Autodesk Inventor part; units mm, degrees
ref_plane "YZ Plane" through (0, 0, 0) normal (1, 0, 0) x (0, 1, 0)
ref_plane "XZ Plane" through (0, 0, 0) normal (0, 1, 0) x (-1, 0, 0)
ref_plane "XY Plane" through (0, 0, 0) normal (0, 0, 1) x (1, 0, 0)
sketch "Sketch1" plane through (0, 0, 0) normal (0, 1, 0) x (-1, 0, 0)
  line L0 (3.175, -63.5) -> (-3.175, -63.5)
  line L1 (-3.175, -63.5) -> (-3.175, 63.5)
  line L2 (-3.175, 63.5) -> (3.175, 63.5)
  line L3 (3.175, 63.5) -> (3.175, -63.5)
  line L4 (3.175, -63.5) -> (-3.175, 63.5) construction
  line L5 (-3.175, -63.5) -> (3.175, 63.5) construction
  circle A0 centre (0, 60.325) radius 2.1082
  circle A1 centre (0, -60.325) radius 2.1082
  point P0 (0, 0)
  dimension "d0" = 6.35
  dimension "d1" = 127
  dimension "d2" = 4.2164
  dimension "d3" = 4.2164
  dimension "d4" = 3.175
  dimension "d5" = 3.175
  dimension "d6" = 3.175
  dimension "d7" = 3.175
extrude "Extrusion1" add sketch "Sketch1" along normal blind 6.35
fillet "Fillet1" radius 1.5875 4 edges at (3.175, 0, 0) (-3.175, 0, 0) (3.175, 6.35, 0) (-3.175, 6.35, 0)
fillet "Fillet2" radius 0.7937 16 edges at (0, 6.35, -63.5) (-2.71, 5.885, -63.5) (-3.175, 3.175, -63.5) (-2.71, 0.465, -63.5) (0, 0, -63.5) (2.71, 0.465, -63.5) (3.175, 3.175, -63.5) (2.71, 5.885, -63.5) (2.71, 5.885, 63.5) (0, 6.35, 63.5) (-2.71, 5.885, 63.5) (-3.175, 3.175, 63.5) (-2.71, 0.465, 63.5) (0, 0, 63.5) (2.71, 0.465, 63.5) (3.175, 3.175, 63.5)
properties part number "cata Beam" material "Stainless Steel"
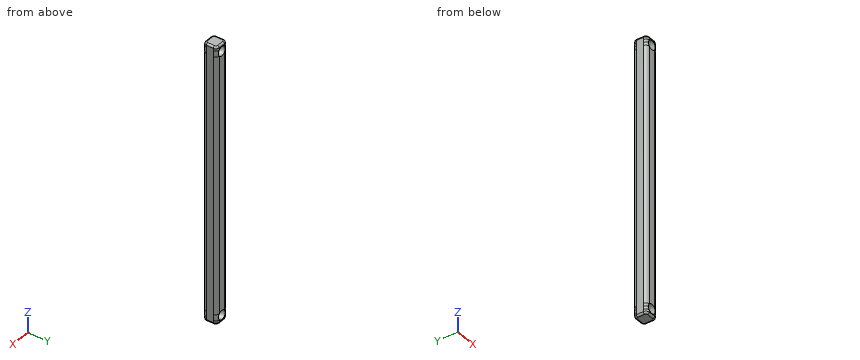
Work out the finished part from the listing and answer in its coordinate system (mm). Give positions to 0.01 mm unless a question says otherwise; leave off trailing zeros. Write each loop counter-clockwise with the first axis right and the second up, starting at its lowest first coordinate (ties: lowest second). Pieces come first, ordered by that corner, then holes. Notation, with made-up numbers: (27.5, 46) -> (46.5, 46) arc R4 ccw to (46.5, 52) -> close; hole circle Ø9 at (88.25, 84.25). An arc over 180 degrees is marked (long way). Write item = value, one per line.
Q1. Consider line 1 along Z through (x, y) = (0, 4.5); line 2 along Z through (x, y) = (-1.25, 0.75); line 3 along Z through (x, y) = (-2.5, 3.5). Determine where each line is inside the solid, lowest interval first.
Computed values:
line_1 = -63.5 to -62.43, -58.22 to 58.22, 62.43 to 63.5
line_2 = -63.5 to -62.02, -58.63 to 58.63, 62.02 to 63.5
line_3 = -63.49 to 63.49
Q2. Section A-A on x = 0 is taken. Determine the outline of the cut face in (y, z), and give its area (3 significant figures).
Computed values:
outline = (0, -62.71) arc R0.79 ccw to (0.79, -63.5) -> (5.56, -63.5) arc R0.79 ccw to (6.35, -62.71) -> (6.35, -62.43) -> (0, -62.43) -> close; (0, -58.22) -> (6.35, -58.22) -> (6.35, 58.22) -> (0, 58.22) -> close; (0, 62.43) -> (6.35, 62.43) -> (6.35, 62.71) arc R0.79 ccw to (5.56, 63.5) -> (0.79, 63.5) arc R0.79 ccw to (0, 62.71) -> close
area = 752 mm^2
Q3. Section B-B on y = 3 is taken. Determine the outline of the cut face in (x, z) (3 decimals), and give its area (3 significant figures).
Computed values:
outline = (-3.175, -62.706) arc R0.794 ccw to (-2.381, -63.5) -> (2.381, -63.5) arc R0.794 ccw to (3.175, -62.706) -> (3.175, 62.706) arc R0.794 ccw to (2.381, 63.5) -> (-2.381, 63.5) arc R0.794 ccw to (-3.175, 62.706) -> close; hole circle Ø4.216 at (0, -60.325); hole circle Ø4.216 at (0, 60.325)
area = 778 mm^2
